```python
from build123d import *

# Parameters (mm, degrees)
REVOLVE8_ANGLE      = 180
SKETCH5_W           = 2.85
SKETCH5_H           = 4.85
BOSS_EXTRUDE1_DEPTH = 2
SKETCH6_W           = 3
SKETCH6_H           = 5
CUT_EXTRUDE1_DEPTH  = 2
FILLET1_R           = 1
SKETCH7_R           = 3.1
CUT_EXTRUDE2_DEPTH  = 40


with BuildPart() as part:
    # Sketch3 → Revolve8 (revolve)
    with BuildSketch(Plane.XY):
        with BuildLine():
            Line((-28.127877823, 11.200453936), (-37.127877823, 61.200453936))
            Line((-37.127877823, 61.200453936), (-39.127877823, 61.200453936))
            Line((-39.127877823, 61.200453936), (-39.127877823, -13.799546064))
            Line((-39.127877823, -13.799546064), (-25.829212511, -13.799546064))
            ThreePointArc((-25.829212511, -13.799546064), (-27.397927857, -3.066483557), (-22.838440036, 6.77580121))
            Line((-22.838440036, 6.77580121), (-22.838440036, 11.200453936))
            Line((-22.838440036, 11.200453936), (-28.127877823, 11.200453936))
        make_face()
    revolve(axis=Axis((-9.127877823, 95.858464184, 0), (0, -1, 0)), revolution_arc=REVOLVE8_ANGLE)

    # Sketch5 → Boss-Extrude1 (add)
    with BuildSketch(Plane.XY):
        with Locations((16.447122177, 13.700453936)):
            Rectangle(SKETCH5_W, SKETCH5_H)
    extrude(amount=BOSS_EXTRUDE1_DEPTH)

    # Sketch6 → Cut-Extrude1 (cut)
    with BuildSketch(Plane.XY):
        with Locations((-34.627877823, 13.700453936)):
            Rectangle(SKETCH6_W, SKETCH6_H)
    extrude(amount=-CUT_EXTRUDE1_DEPTH, mode=Mode.SUBTRACT)

    # Fillet1
    fillet1_edges = [part.edges().sort_by_distance(p)[0] for p in [
        (-9.127877823, -13.799546064, -16.701334688),
    ]]
    fillet(fillet1_edges, radius=FILLET1_R)

    # Sketch7 → Cut-Extrude2 (cut)
    with BuildSketch(Plane.XY):
        with Locations((-9.127877823, 23.700453936)):
            Circle(SKETCH7_R)
        with Locations((-9.127877823, 48.700453936)):
            Circle(SKETCH7_R)
    extrude(amount=-CUT_EXTRUDE2_DEPTH, mode=Mode.SUBTRACT)


solid = part.part
```
Build history of the part. All positions in model axes, mm. A direction names the side the tool comes from. Coordinates: 2 decimals unless noted, no trailing zeros. Write each loop counter-clockwise with the first axis right and the second up, starting at its lowest first coordinate (ties: lowest second). Pieces come first, ordered by that corner, then holes.
1. Band-saw the part on B-B, the plane x = -10.5. Give the number of separate pieces and of enclosed holes in the cut face, and give its area (3 significant figures).
Answer block:
separate pieces: 3
enclosed holes: 0
area: 586 mm2
2. 3-axis set-ups, long thin cutter, end or side, ignore diameter. For faces 1 (the flat face through (-33.128, 14, -1)), 2 (the flat face through (16, 11.275, 1)), 3 (the flat face through (15.022, 14, 1)), 4 (the flat face through (16, 16.125, 1)): which of +Z, -Z, +X, -X, +Y, -Y reach the whole face in a straight line?
Answer block:
face 1: +Z
face 2: +Z, +X, -X, -Y
face 3: +Z, -X, +Y, -Y
face 4: +Z, +X, -X, +Y
3. Drop flat-ended pins along their axis: pin 1 (6 mm diameter, centred on y = 18.5, z = -8, fed in from -X); pin 2 (5 mm diameter, centred on y = 15.5, z = -6, fed in from +X); pin 3 (5 mm diameter, centred on y = 15, z = -2.5, fed in from +X); pin 4 (5 mm diameter, centred on x = -28, y = 19.5, fed in from -Z). Give the stop position or say it passes through.
Answer block:
pin 1: stops at x = -38.71
pin 2: stops at x = 20.67
pin 3: stops at x = 20.87
pin 4: stops at z = -25.14
4. Band-saw the part on A-A, the plane y = 13.5. Give the cut face in (x, z), and give its area (3 significant figures).
Answer block:
outline: (-39.13, 0) arc R30 ccw to (20.87, 0) - (17.87, 0) - (17.87, 2) - (15.02, 2) - (15.02, 0) - (10.29, 0) arc R19.41 cw to (-28.54, 0) - (-33.13, 0) - (-33.13, -2) - (-36.13, -2) - (-36.13, 0) - close
area: 821 mm2
5. Drill centre lines: probe 1 along X at (y, z) = (26, -26.5); probe 2 along X at (y, z) = (10.5, -8.5); probe 3 along X at (y, z) = (9, -18). Where is each one in solid material? Low to high.
Answer block:
probe 1: x = -23.19 to -11.21, -7.05 to 4.93
probe 2: x = -37.9 to -19.89, 1.63 to 19.64
probe 3: x = -33.13 to 14.87
6. Pull direction X, two halves, no side cores. Call faces 5 (the flat face through (-9, 11.2, -14)), 6 (the flat face through (-35, 16.2, -1)), 7 (the cylindrical face through (-9.788, 14.842, -29.993)), 8 (the flat face through (-9.3, 61.2, -28.4)): released by +X, released by -X, zero draft, split by the parting line, or undercut.
Answer block:
face 5: undercut
face 6: undercut
face 7: split by the parting line
face 8: zero draft
